Part print with two shaded views. Sizes in mm from the minimum x, y, z corner. Round coordinates to 2 decimals unless told otherwise and drop trailing zeros. Loops run counter-clockwise (first coordinate to the right, second up) from the corner with the lowest first, then second, coordinate; pieces in that order, holes last. Notation, with made-up numbers: (60, 26.5) -> (66, 26.5) arc R22 cw to (66, 52.5) -> close; hole circle Ø11 at (3, -31). An arc over 180 degrees is marked (long way). Use a Markdown table: item, result. Add a question column.
Item 1: Cut at B-B, the plane z = 8. List the corners of the cut face in (x, y).
Item 2: Cut at D-D, the plane x = 74.5. List the corners of the cut face in (y, z), plus the area to 3 significant figures.
Item 3: Probe line 1 (X direction, y = 0.75, z = 5); line 2 (Z direction, x = 115, y = 0.7); line 3 (Z direction, x = 65, y = 13.75). List the from-to ranges inside material, lowest first. Write a range as [from, to].
Item 4: Cut at C-C, the plane x = 5. List the corners of the cut face in (y, z).
Item 5: Cut at A-A, the plane y = 6.25. List the corners of the cut face in (x, z).
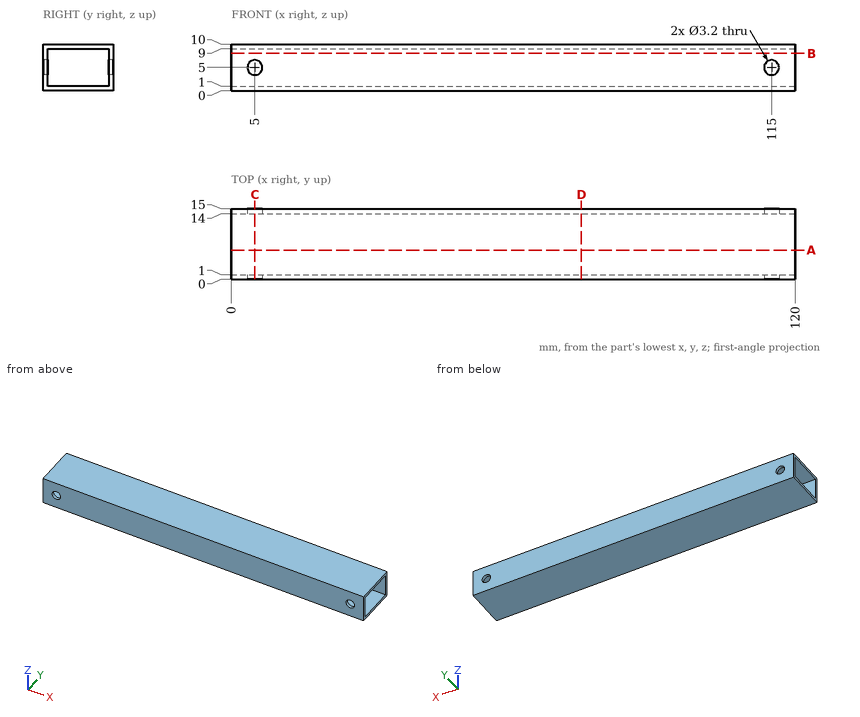
A:
| question | item | result |
|---|---|---|
| 1 | outline | (0, 0) -> (120, 0) -> (120, 1) -> (0, 1) -> close; (0, 14) -> (120, 14) -> (120, 15) -> (0, 15) -> close |
| 2 | outline | (0, 0) -> (15, 0) -> (15, 10) -> (0, 10) -> close; hole (1, 1) -> (14, 1) -> (14, 9) -> (1, 9) -> close |
| 2 | area | 46.0 mm^2 |
| 3 | line 1 | x = [0, 3.4], [6.6, 113.4], [116.6, 120] |
| 3 | line 2 | z = [0, 3.4], [6.6, 10] |
| 3 | line 3 | z = [0, 1], [9, 10] |
| 4 | outline | (0, 0) -> (15, 0) -> (15, 3.4) -> (14, 3.4) -> (14, 1) -> (1, 1) -> (1, 3.4) -> (0, 3.4) -> close; (0, 6.6) -> (1, 6.6) -> (1, 9) -> (14, 9) -> (14, 6.6) -> (15, 6.6) -> (15, 10) -> (0, 10) -> close |
| 5 | outline | (0, 0) -> (120, 0) -> (120, 1) -> (0, 1) -> close; (0, 9) -> (120, 9) -> (120, 10) -> (0, 10) -> close |
